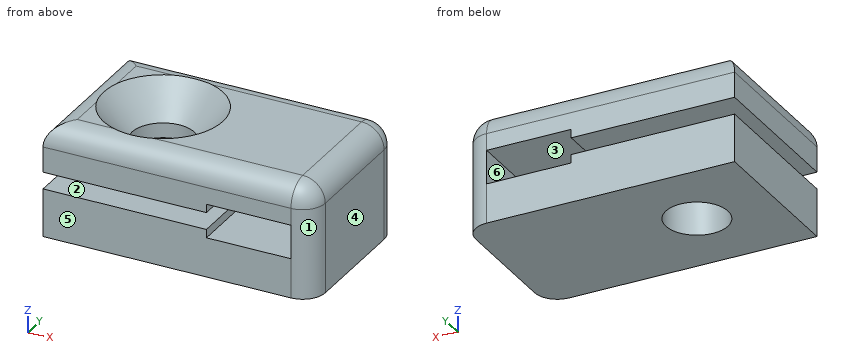
from build123d import *

# Parameters (mm, degrees)
F0_W           = 5
F0_H           = 7
F0_W_2         = 7
F1_DEPTH       = 5
F3_D           = 2.75
F3_CSINK_D     = 5.3
F3_CSINK_ANGLE = 82
F5_DEPTH       = 7
F6_T1_DEPTH    = 12
F6_T3_DEPTH    = 13.5
F6_T5_DEPTH    = 5
F6_T7_DEPTH    = 6.5
F6_S11_W       = 1
F6_S11_H       = 1
F6_T12_DEPTH   = 1
F6_S17_W       = 1
F6_S17_H       = 1
F6_T18_DEPTH   = 1


# Not quite as in the source:
# - a fillet or chamfer that OpenCascade refuses, or shapes differently, is made with other operations: its cross-section is extruded or revolved along the edge and cut away or added


with BuildPart() as f1:
    # F0 (on Top) → F1 (new body)
    with BuildSketch(Plane.XY):
        with Locations((3.5, 0)):
            Rectangle(F0_W, F0_H)
        with Locations((-2.5, 0)):
            Rectangle(F0_W_2, F0_H)
    extrude(amount=-F1_DEPTH)

    # F3 (through all)
    with Locations(Plane.XY):
        with Locations((-2.5, 0)):
            CounterSinkHole(F3_D / 2, F3_CSINK_D / 2, counter_sink_angle=F3_CSINK_ANGLE)

    # F4 (on face) → F5 (cut, through all)
    with BuildSketch(Plane.XZ.offset(3.5)):
        Polygon((1.25, -3.25), (4.9999998882, -3.25), (4.9999998882, -1.75), (1.25, -1.75), (1.25, -2.125), (-6, -2.125), (-6, -2.875), (1.25, -2.875), align=None)
    extrude(amount=-F5_DEPTH, mode=Mode.SUBTRACT)

    # F6: fillet of radius 1 on 6 edges, made by hand

    # F6_s2 → F6_t1 (cut)
    with BuildSketch(Plane.XZ.offset(-6)):
        with BuildLine():
            ThreePointArc((-5, 0), (-5.7071067812, -0.2928932188), (-6, -1))
            Line((-6, -1), (-6, 0))
            Line((-6, 0), (-5, 0))
        make_face()
    extrude(amount=F6_T1_DEPTH, mode=Mode.SUBTRACT)

    # F6_s4 → F6_t3 (cut)
    with BuildSketch(Plane.YZ.offset(-8.5)):
        with BuildLine():
            ThreePointArc((3.5, -1), (3.2071067812, -0.2928932188), (2.5, 0))
            Line((2.5, 0), (3.5, 0))
            Line((3.5, 0), (3.5, -1))
        make_face()
        with BuildLine():
            ThreePointArc((-3.5, -1), (-3.2071067812, -0.2928932188), (-2.5, 0))
            Line((-2.5, 0), (-3.5, 0))
            Line((-3.5, 0), (-3.5, -1))
        make_face()
    extrude(amount=F6_T3_DEPTH, mode=Mode.SUBTRACT)

    # F6_s6 → F6_t5 (cut)
    with BuildSketch(Plane.XZ.offset(-2.5)):
        with BuildLine():
            ThreePointArc((6, -1), (5.7071067812, -0.2928932188), (5, 0))
            Line((5, 0), (6, 0))
            Line((6, 0), (6, -1))
        make_face()
    extrude(amount=F6_T5_DEPTH, mode=Mode.SUBTRACT)

    # F6_s8 → F6_t7 (cut)
    with BuildSketch(Plane.XY.offset(-7.5)):
        with BuildLine():
            ThreePointArc((6, -2.5), (5.7071067812, -3.2071067812), (5, -3.5))
            Line((5, -3.5), (6, -3.5))
            Line((6, -3.5), (6, -2.5))
        make_face()
        with BuildLine():
            ThreePointArc((6, 2.5), (5.7071067812, 3.2071067812), (5, 3.5))
            Line((5, 3.5), (6, 3.5))
            Line((6, 3.5), (6, 2.5))
        make_face()
    extrude(amount=F6_T7_DEPTH, mode=Mode.SUBTRACT)


with BuildPart() as f6_tool10:
    # F6_s11 → F6_t12 (new body)
    with BuildSketch(Plane.YZ.offset(5)):
        with Locations((3, -0.5)):
            Rectangle(F6_S11_W, F6_S11_H)
    extrude(amount=F6_T12_DEPTH)

    # F6_s13 → F6_t14 (revolve, cut)
    with BuildSketch(Plane(origin=(5, 2.5, -1), x_dir=(0, -0.7071067812, -0.7071067812), z_dir=(0, -0.7071067812, 0.7071067812))):
        with BuildLine():
            ThreePointArc((0, -1), (1, 0), (0, 1))
            Line((0, 1), (0, -1))
        make_face()
    revolve(axis=Axis((5, 2.5, -1), (1, 0, 0)), mode=Mode.SUBTRACT)


with BuildPart() as f1_1:
    add(f1.part)

    # F6_t9: cut F6_tool10
    add(f6_tool10.part, mode=Mode.SUBTRACT)


with BuildPart() as f6_tool16:
    # F6_s17 → F6_t18 (new body)
    with BuildSketch(Plane.YZ.offset(5)):
        with Locations((-3, -0.5)):
            Rectangle(F6_S17_W, F6_S17_H)
    extrude(amount=F6_T18_DEPTH)

    # F6_s19 → F6_t20 (revolve, cut)
    with BuildSketch(Plane(origin=(5, -2.5, -1), x_dir=(0, 0.7071067812, -0.7071067812), z_dir=(0, -0.7071067812, -0.7071067812))):
        with BuildLine():
            ThreePointArc((0, -1), (1, 0), (0, 1))
            Line((0, 1), (0, -1))
        make_face()
    revolve(axis=Axis((5, -2.5, -1), (1, 0, 0)), mode=Mode.SUBTRACT)


with BuildPart() as f1_2:
    add(f1_1.part)

    # F6_t15: cut F6_tool16
    add(f6_tool16.part, mode=Mode.SUBTRACT)


solid = f1_2.part
CAD build for the part. Positions are in the model's coordinates, mm. Face numbers are marked on the shaded views. A direction names the side the tool comes from. Round coordinates to 2 decimals unless told otherwise and drop trailing zeros. Write each loop counter-clockwise with the first axis right and the second up, starting at its lowest first coordinate (ties: lowest second). Pieces come first, ordered by that corner, then holes.
(1) Slice it at A-A, the plane x = 1.5. Write the cut outline in (y, z), and give its area (3 significant figures).
(2) Slice it at B-B, the plane y = 0. Write the cut outline in (x, z) (3 decimals), and give its area (3 significant figures).
(3) Slice it at D-D, the plane z = -3.4. Write the cut outline in (x, y) (3 decimals).
(4) 3-axis set-ups, long thin cutter, end or side, ignore diameter. For the marked faces 1, 2 and 3: which of +Z, -Z, +X, -X, +Y, -Y reach the whole face in a straight line?
(5) Drop flat-ended pins along their axis: P1, Ø2, axis at x = -2.5, y = 0, coming from the -Z side; P2, Ø4, axis at x = 3.5, y = 1.5, coming from the +Z side. Give the stop position or say it passes through.
(6) Mould opens along X. For the marked faces 4, 5 and 6 say: pulls with the +X half, pulls with the -X half, needs draft (parallel to the pull), parting line crosses it, or undercut.
(7) Slice it at C-C, the plane x = -2.5. Write the cut outline in (y, z) (3 decimals).
(8) Probe line 1 along Y through (x, z) = (-2.5, -3.5) (3 decimals); line 2 along Z through (x, y) = (2.75, 1); line 3 along Z through (x, y) = (0, -2.5) (3 decimals). List the from-to ranges inside material, lowest first.
From the geometry:
1. outline: (-3.5, -5) - (3.5, -5) - (3.5, -3.25) - (-3.5, -3.25) - close; (-3.5, -1.75) - (3.5, -1.75) - (3.5, -1) arc R1 ccw to (2.5, 0) - (-2.5, 0) arc R1 ccw to (-3.5, -1) - close
1. area: 24.1 mm2
2. outline: (-6, -5) - (-3.875, -5) - (-3.875, -2.875) - (-6, -2.875) - close; (-6, -2.125) - (-3.875, -2.125) - (-3.875, -1.467) - (-5.141, -0.01) arc R1 ccw to (-6, -1) - close; (-1.125, -5) - (6, -5) - (6, -1) arc R1 ccw to (5, 0) - (0.15, 0) - (-1.125, -1.467) - (-1.125, -2.125) - (1.25, -2.125) - (1.25, -1.75) - (5, -1.75) - (5, -3.25) - (1.25, -3.25) - (1.25, -2.875) - (-1.125, -2.875) - close
2. area: 35.0 mm2
3. outline: (-6, -3.5) - (5, -3.5) arc R1 ccw to (6, -2.5) - (6, 2.5) arc R1 ccw to (5, 3.5) - (-6, 3.5) - close; hole circle Ø2.75 at (-2.5, 0)
4. face 1: +Z, -Z, +X, -Y
4. face 2: -X, +Y, -Y
4. face 3: +Y, -Y
5. P1: passes through
5. P2: stops at z = 0
6. face 4: pulls with the +X half
6. face 5: needs draft
6. face 6: undercut
7. outline: (-3.5, -5) - (-1.375, -5) - (-1.375, -2.875) - (-3.5, -2.875) - close; (-3.5, -2.125) - (-1.375, -2.125) - (-1.375, -1.467) - (-2.641, -0.01) arc R1 ccw to (-3.5, -1) - close; (1.375, -5) - (3.5, -5) - (3.5, -2.875) - (1.375, -2.875) - close; (1.375, -2.125) - (3.5, -2.125) - (3.5, -1) arc R1 ccw to (2.641, -0.01) - (1.375, -1.467) - close
8. line 1: y = -3.5 to -1.375, 1.375 to 3.5
8. line 2: z = -5 to -3.25, -1.75 to 0
8. line 3: z = -5 to -2.875, -2.125 to 0
